Here's how the part is built. I have some questions about the finished solid (model axes, mm). Face numbers are marked on the shaded views. A direction names the side the tool comes from. Give positions to 0.01 mm unless a question says otherwise; leave off trailing zeros. Order: outer loops, then holes, each group sorted by start corner. A loop starts at its lowest first (then second) coordinate and runs counter-clockwise, first axis right, second up.
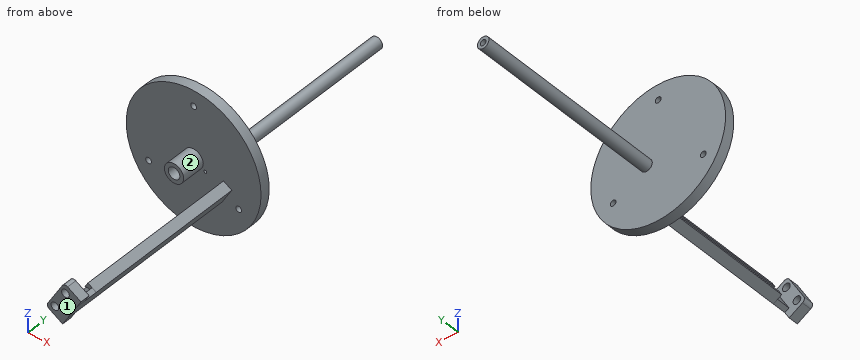
from build123d import *

# Parameters (mm, degrees)
F0_R      = 35
F1_DEPTH  = 5
F2_R      = 5
F2_R_2    = 3
F3_DEPTH  = 12
F5_DEPTH  = 83
F7_D      = 3
F7_DEPTH  = 6
F7_TIP    = 0.9012909285
F9_DEPTH  = 83
F10_R     = 3
F11_DEPTH = 6.5
F13_DEPTH = 7
F15_DEPTH = 5
F17_D     = 4
F17_DEPTH = 10
F17_TIP   = 1.2017212381
F19_D     = 1.5
F19_DEPTH = 10
F19_TIP   = 0.4506454643
F20_R     = 3
F20_R_2   = 1.5
F21_DEPTH = 100


# Not quite as in the source:
# - a feature names something its author has since deleted; it is built from what else it names


with BuildPart() as f1:
    # F0 (on Front) → F1 (new body)
    with BuildSketch(Plane.XZ):
        Circle(F0_R)
    extrude(amount=F1_DEPTH)

    # F2 (on face) → F3 (join)
    with BuildSketch(Plane.XZ.offset(5)):
        Circle(F2_R)
        Circle(F2_R_2, mode=Mode.SUBTRACT)
    extrude(amount=F3_DEPTH)

    # F4 (on face) → F5 (join)
    with BuildSketch(Plane.XZ.offset(5)):
        Polygon((14.8205080757, -14.3301270189), (19.8205080757, -5.6698729811), (15.4903810568, -3.1698729811), (10.4903810568, -11.8301270189), align=None)
    extrude(amount=F5_DEPTH)

    # F7
    with Locations(Plane(origin=(0, 0, 0), x_dir=(-1, 0, 0), z_dir=(0, 1, 0))):
        with Locations((0, 27), (-23.3826859022, -13.5), (23.3826859022, -13.5)):
            Hole(F7_D / 2, depth=F7_DEPTH)
            with Locations((0, 0, -(F7_DEPTH + F7_TIP / 2))):  # 118° drill point
                Cone(0, F7_D / 2, F7_TIP, mode=Mode.SUBTRACT)

    # F8 (on face) → F9 (cut, through all)
    with BuildSketch(Plane.XZ.offset(88)):
        with BuildLine():
            Line((13.9903810568, -5.7679491924), (11.9903810568, -9.2320508076))
            Line((11.9903810568, -9.2320508076), (13.0007440278, -10.9820508076))
            ThreePointArc((13.0007440278, -10.9820508076), (13.4337567297, -11.2320508076), (13.8667694316, -10.9820508076))
            Line((13.8667694316, -10.9820508076), (16.4441197008, -6.5179491924))
            ThreePointArc((16.4441197008, -6.5179491924), (16.4441197008, -6.0179491924), (16.0111069989, -5.7679491924))
            Line((16.0111069989, -5.7679491924), (13.9903810568, -5.7679491924))
        make_face()
    extrude(amount=-F9_DEPTH, mode=Mode.SUBTRACT)

    # F10 (on face) → F11 (join)
    with BuildSketch(Plane.XZ.offset(5)):
        Circle(F10_R)
    extrude(amount=F11_DEPTH)

    # F12 (on face) → F13 (join)
    with BuildSketch(Plane.XZ.offset(88)):
        Polygon((12.6554445662, -13.0801270189), (14.8205080757, -14.3301270189), (19.8205080757, -5.6698729811), (17.6554445662, -4.4198729811), align=None)
    extrude(amount=F13_DEPTH)

    # F14 (on face) → F15 (join)
    with BuildSketch(Plane.XZ.offset(95)):
        with BuildLine():
            Line((5.6423048454, -14.227241336), (12.5705080757, -18.227241336))
            Line((12.5705080757, -18.227241336), (14.8205080757, -14.3301270189))
            Line((14.8205080757, -14.3301270189), (12.6554445662, -13.0801270189))
            Line((12.6554445662, -13.0801270189), (17.6554445662, -4.4198729811))
            Line((17.6554445662, -4.4198729811), (19.8205080757, -5.6698729811))
            Line((19.8205080757, -5.6698729811), (22.0705080757, -1.772758664))
            Line((22.0705080757, -1.772758664), (15.1423048454, 2.227241336))
            ThreePointArc((15.1423048454, 2.227241336), (13.6246667552, 2.427042181), (12.4102540378, 1.4951905284))
            Line((12.4102540378, 1.4951905284), (4.9102540378, -11.4951905284))
            ThreePointArc((4.9102540378, -11.4951905284), (4.7104531928, -13.0128286186), (5.6423048454, -14.227241336))
        make_face()
        Polygon((12.6554445662, -13.0801270189), (14.8205080757, -14.3301270189), (19.8205080757, -5.6698729811), (17.6554445662, -4.4198729811), align=None)
    extrude(amount=F15_DEPTH)

    # F17
    with Locations(Plane.XZ.offset(100)):
        with Locations((14.0083302492, -1.7368602792), (8.5083302492, -11.2631397208)):
            Hole(F17_D / 2, depth=F17_DEPTH)
            with Locations((0, 0, -(F17_DEPTH + F17_TIP / 2))):  # 118° drill point
                Cone(0, F17_D / 2, F17_TIP, mode=Mode.SUBTRACT)

    # F19
    with Locations(Plane.XZ.offset(5)):
        with Locations((6.0621778265, -3.5)):
            Hole(F19_D / 2, depth=F19_DEPTH)
            with Locations((0, 0, -(F19_DEPTH + F19_TIP / 2))):  # 118° drill point
                Cone(0, F19_D / 2, F19_TIP, mode=Mode.SUBTRACT)

    # F20 (on face) → F21 (join)
    with BuildSketch(Plane(origin=(0, 0, 0), x_dir=(-1, 0, 0), z_dir=(0, 1, 0))):
        with Locations((-6.0621778265, -3.5)):
            Circle(F20_R)
        with Locations((-6.0621778265, -3.5)):
            Circle(F20_R_2, mode=Mode.SUBTRACT)
    extrude(amount=F21_DEPTH)


solid = f1.part
Q1. If we section it at A-A on y = -13.5: List the corners of the cut face in (x, z) for me.
Filled sheet:
outline: circle Ø10 at (0, 0); (10.49, -11.83) - (14.82, -14.33) - (19.82, -5.67) - (15.49, -3.17) - (13.99, -5.77) - (16.01, -5.77) arc R0.5 cw to (16.44, -6.52) - (13.87, -10.98) arc R0.5 cw to (13, -10.98) - (11.99, -9.23) - close; hole circle Ø6 at (0, 0)
Q2. For the marked faces 1 and 2, which set-ups out of +Z, -Z, +X, -X, +Y, -Y let a thin tool reach every point of the face, with its end or its side?
Filled sheet:
face 1: +Z, -Z, +X, -X, -Y
face 2: -Y
Q3. If we section it at C-C on z = 10.5: List the corners of the cut face in (x, y) for me, plus the area to 3 significant figures.
Filled sheet:
outline: (-33.39, -5) - (33.39, -5) - (33.39, 0) - (-33.39, 0) - close
area: 334 mm2
Q4. If we section it at D-D on x = 30: List the corners of the cut face in (y, z) for me, plus the area to 3 significant figures.
Filled sheet:
outline: (-5, -18.03) - (0, -18.03) - (0, 18.03) - (-5, 18.03) - close
area: 180 mm2
Q5. I need wall thicknesses on L1, parallel to Y at x = 29, z = 15.5; L2, parallel to X at y = -0.5, z = -29; L3, parallel to Z at x = 15.5, y = -20.5. Which ranges of each line are inside material? Lowest first, please.
Filled sheet:
L1: y = -5 to 0
L2: x = -19.6 to 19.6
L3: z = -13.15 to -8.15, -5.77 to -3.18
Q6. If we section it at B-B on y = 52.5: List the corners of the cut face in (x, z) for me.
Filled sheet:
outline: circle Ø6 at (6.06, -3.5); hole circle Ø3 at (6.06, -3.5)
Q7. I'm going to push flat-ended pins straight in: P1, Ø5, axis at y = 40.5, z = -0.5, coming from the -X side; P2, Ø6.5, axis at x = 14.01, z = -1.74, coming from the +Y side; P3, Ø5, axis at x = 20, y = -9.5, coming from the +Z side. Where does each tip first touch, or does it pass through?
Filled sheet:
P1: stops at x = 3.1
P2: stops at y = 0
P3: stops at z = -4.33
